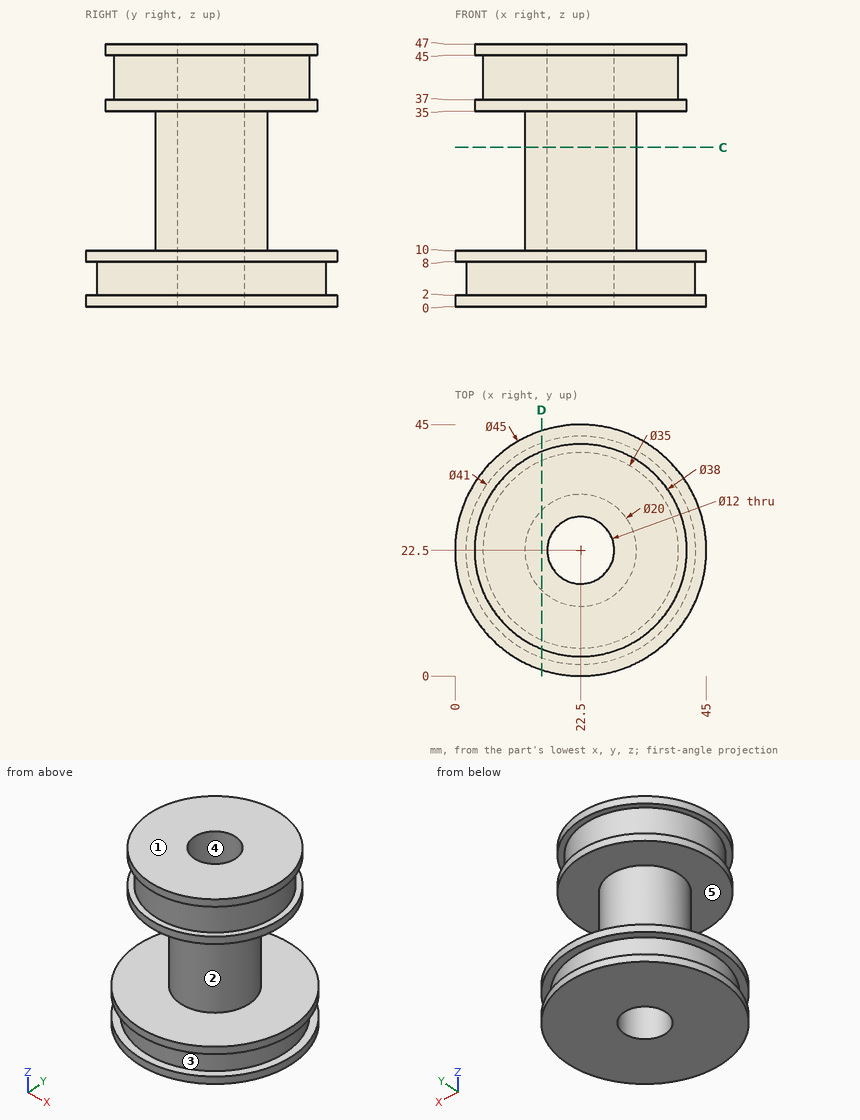
The drawing under review shows one solid part. Ordinate dimensions are in mm from its lowest x, y, z. A direction names the side the tool comes from. Round coordinates to 2 decimals unless told otherwise and drop trailing zeros. Loops run counter-clockwise (first coordinate to the right, second up) from the corner with the lowest first, then second, coordinate; pieces in that order, holes last. Notation, with made-up numbers: (56, 58.5) - (72, 58.5) arc R21 ccw to (72, 83.5) - close; hole circle Ø3 at (73, 84). An arc over 180 degrees is marked (long way). Put each result on its own line as item: value. Start each with the question number.
1. Consider section D-D on x = 15.5. State the section outline as (y, z) points.
2. Insertion check: P1, Ø2, axis at x = 17, z = 29, coming from the +Y side; P2, Ø10, axis at y = 35.5, z = 25.5, coming from the -X side; P3, Ø6, axis at y = 14, z = 24, coming from the -X side. Each pin has a flat end and moves straight along its axis. Give the tip position at first contact, or say it passes through.
3. Consider section C-C on z = 28.5. State the section outline as (x, y) points, plus the area to 3 significant figures.
4. For probe 1 along Z at (x, y) = (39.5, 35.5); probe 2 along Z at (x, y) = (7.5, 34); probe 3 along Z at (x, y) = (33, 29.5), list the stretches that pass through material, from the lowest coordinate up. Write a range as [from, to].
5. For the marked faces 1 and 2, list the 3-axis set-ups (+Z, -Z, +X, -X, +Y, -Y) from which the entire face can be reached by the end or side of a thin tool; tool diameter is ignored.
6. Mouldability with a two-part tool opening along Y and no side actions: class the marked faces 3, 4 and 5 as +Y half, -Y half, draft (parallel to the pull), parting line (faces both ways), or undercut.
Result sheet:
1. outline: (1.12, 0) - (43.88, 0) - (43.88, 2) - (41.77, 2) - (41.77, 8) - (43.88, 8) - (43.88, 10) - (29.64, 10) - (29.64, 35) - (40.16, 35) - (40.16, 37) - (38.54, 37) - (38.54, 45) - (40.16, 45) - (40.16, 47) - (4.84, 47) - (4.84, 45) - (6.46, 45) - (6.46, 37) - (4.84, 37) - (4.84, 35) - (15.36, 35) - (15.36, 10) - (1.12, 10) - (1.12, 8) - (3.23, 8) - (3.23, 2) - (1.12, 2) - close
2. P1: y = 31.43
2. P2: x = 16.5
2. P3: x = 14.15
3. outline: circle Ø20 at (22.5, 22.5); hole circle Ø12 at (22.5, 22.5)
3. area: 201 mm^2
4. probe 1: [0, 2], [8, 10]
4. probe 2: [0, 10], [35, 37], [45, 47]
4. probe 3: [0, 10], [35, 47]
5. face 1: +Z, +X, -X, +Y, -Y
5. face 2: none
6. face 3: parting line
6. face 4: undercut
6. face 5: draft
